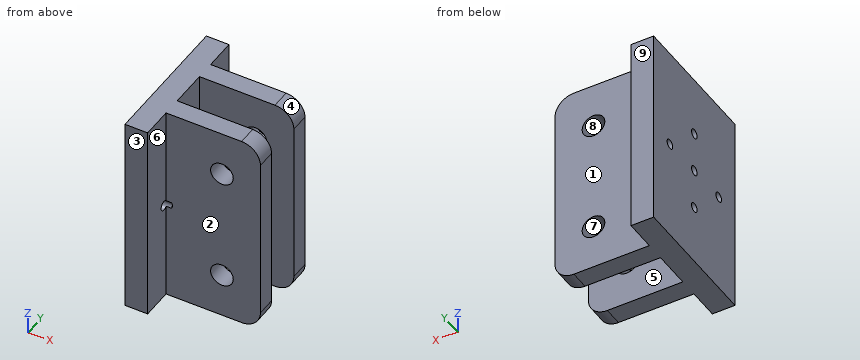
```python
from build123d import *

# Parameters (mm, degrees)
SKETCH_1_W             = 53.8
SKETCH_1_H             = 36.5
EXTRUDE_1_DEPTH        = 6
SKETCH_2_W             = 53.8
SKETCH_2_H             = 20
EXTRUDE_2_DEPTH        = 25
SKETCH_3_W             = 53.8
SKETCH_3_H             = 10
CUT_EXTRUDE_1_DEPTH    = 25
HOLE_WIZARD_M3_1_D     = 2.5
HOLE_WIZARD_M3_1_DEPTH = 7.5
HOLE_WIZARD_M3_1_TIP   = 0.751075774
SKETCH_6_R             = 3
CUT_EXTRUDE_2_DEPTH    = 29.25
FILLET_1_R             = 5


with BuildPart() as part:
    # 草图1 → 凸台-拉伸1 (new body)
    with BuildSketch(Plane(origin=(0, 0, 0), x_dir=(0, 0, -1), z_dir=(1, 0, 0))):
        Rectangle(SKETCH_1_W, SKETCH_1_H)
    extrude(amount=EXTRUDE_1_DEPTH)

    # 草图2 → 凸台-拉伸2 (add)
    with BuildSketch(Plane(origin=(6, 0, 0), x_dir=(0, 0, -1), z_dir=(1, 0, 0))):
        Rectangle(SKETCH_2_W, SKETCH_2_H)
    extrude(amount=EXTRUDE_2_DEPTH)

    # 草图3 → 切除-拉伸1 (cut)
    with BuildSketch(Plane(origin=(31, 0, 0), x_dir=(0, 0, -1), z_dir=(1, 0, 0))):
        Rectangle(SKETCH_3_W, SKETCH_3_H)
    extrude(amount=-CUT_EXTRUDE_1_DEPTH, mode=Mode.SUBTRACT)

    # M3 螺纹孔1
    with Locations(Plane.ZY):
        with Locations((-10.95, 0), (0, 10.95), (0, 0), (0, -10.95), (10.95, 0)):
            Hole(HOLE_WIZARD_M3_1_D / 2, depth=HOLE_WIZARD_M3_1_DEPTH)
            with Locations((0, 0, -(HOLE_WIZARD_M3_1_DEPTH + HOLE_WIZARD_M3_1_TIP / 2))):  # 118° drill point
                Cone(0, HOLE_WIZARD_M3_1_D / 2, HOLE_WIZARD_M3_1_TIP, mode=Mode.SUBTRACT)

    # 草图6 → 切除-拉伸2 (cut, through all)
    with BuildSketch(Plane.XZ.offset(10)):
        with Locations((20.806055882, 15)):
            Circle(SKETCH_6_R)
        with Locations((20.806055882, -15)):
            Circle(SKETCH_6_R)
    extrude(amount=-CUT_EXTRUDE_2_DEPTH, mode=Mode.SUBTRACT)

    # 圆角1
    fillet_1_edges = [part.edges().sort_by_distance(p)[0] for p in [
        (31, -7.5, -26.9),
        (31, 7.5, 26.9),
        (31, 7.5, -26.9),
        (31, -7.5, 26.9),
    ]]
    fillet(fillet_1_edges, radius=FILLET_1_R)


solid = part.part
```
Model file for the job. Use its own axes, mm. Face numbers are marked on the shaded views. A direction names the side the tool comes from. Give positions to 0.01 mm unless a question says otherwise; leave off trailing zeros. Write each loop counter-clockwise with the first axis right and the second up, starting at its lowest first coordinate (ties: lowest second). Pieces come first, ordered by that corner, then holes. Notation, with made-up numbers: (-40, -8) - (15, -8) arc R24 cw to (15, 15) - close; hole circle Ø5 at (62.5, -36.75). An arc over 180 degrees is marked (long way). One line per question, with ' | ' between items. Start each with the question number.
(1) Slice it at B-B on z = 0. Write the cut outline in (x, y), plus the area to 3 significant figures.
(2) Wall check: line 1 along Z through (x, y) = (1.75, -10.95); line 2 along Y through (x, z) = (7, -20.5); line 3 along Y through (x, z) = (2.55, 10.95). Give the ranges that are in metal, low to high. Write a range as from..to.
(3) Pin check, flat tips, straight feed: P1, Ø2, axis at y = 10.95, z = 0, coming from the -X side; P2, Ø5, axis at y = 2, z = -7.5, coming from the +X side; P3, Ø5.5, axis at x = 20.81, z = -15, coming from the +Y side; P4, Ø1, axis at x = 9, z = 18.5, coming from the +Y side. Stop position of each tip, or through.
(4) Two-plate mould, pull along X, no slides. Class the marked faces 6, 7, 8 and 9: +X half, -X half, draft (parallel to the pull), parting line (faces both ways), or undercut.
(5) Slice it at D-D on y = 6.5. Write the cut outline in (x, z), plus the area to 3 significant figures.
(6) Slice it at A-A on x = 29. Write the cut outline in (y, z), plus the area to 3 significant figures.
(7) 3-axis set-ups, long thin cutter, end or side, ignore diameter. For the marked faces 1, 2, 3, 4 and 5: which of +Z, -Z, +X, -X, +Y, -Y reach the whole face in a straight line?
(8) Slice it at C-C on z = -15. Write the cut outline in (x, y).
Results below:
1) outline: (0, -18.25) - (6, -18.25) - (6, -12.2) - (0, -12.2) - close; (0, -9.7) - (7.5, -9.7) - (7.68, -10) - (31, -10) - (31, -5) - (6, -5) - (6, -1.25) - (0, -1.25) - close; (0, 1.25) - (6, 1.25) - (6, 5) - (31, 5) - (31, 10) - (7.68, 10) - (7.5, 9.7) - (0, 9.7) - close; (0, 12.2) - (6, 12.2) - (6, 18.25) - (0, 18.25) - close | area: 423 mm^2
2) line 1: -26.9..-1.25, 1.25..26.9 | line 2: -10..-5, 5..10 | line 3: -18.25..-1.25, 1.25..18.25
3) P1: x = 7.65 | P2: x = 6 | P3: through | P4: y = 10
4) face 6: +X half | face 7: undercut | face 8: undercut | face 9: draft
5) outline: (0, -26.9) - (26, -26.9) arc R5 ccw to (31, -21.9) - (31, 21.9) arc R5 ccw to (26, 26.9) - (0, 26.9) - close; hole circle Ø6 at (20.81, -15); hole circle Ø6 at (20.81, 15) | area: 1,600 mm^2
6) outline: (-10, -25.9) - (-5, -25.9) - (-5, 25.9) - (-10, 25.9) - close; (5, -25.9) - (10, -25.9) - (10, 25.9) - (5, 25.9) - close | area: 518 mm^2
7) face 1: +Z, -Z, +X, +Y | face 2: +Z, -Z, +X, -Y | face 3: +Z, -Z, +X, -X, -Y | face 4: +Z, +X, +Y, -Y | face 5: +Z, -Z, +X
8) outline: (0, -18.25) - (6, -18.25) - (6, -10) - (17.81, -10) - (17.81, -5) - (6, -5) - (6, 5) - (17.81, 5) - (17.81, 10) - (6, 10) - (6, 18.25) - (0, 18.25) - close; (23.81, -10) - (31, -10) - (31, -5) - (23.81, -5) - close; (23.81, 5) - (31, 5) - (31, 10) - (23.81, 10) - close
